from build123d import *

# Parameters (mm, degrees)
SKETCH1_R           = 11.2
BOSS_EXTRUDE1_DEPTH = 232.947291788
CUT_EXTRUDE1_DEPTH  = 236.982


with BuildPart() as part:
    # Sketch1 → Boss-Extrude1 (new body)
    with BuildSketch(Plane.XY):
        with BuildLine():
            Line((-25.4, -67.479999962), (-25.4, 36.365))
            ThreePointArc((-25.4, 36.365), (-23.726115254, 40.406115254), (-19.685, 42.08))
            Line((-19.685, 42.08), (32.385, 42.08))
            ThreePointArc((32.385, 42.08), (36.426115254, 40.406115254), (38.1, 36.365))
            Line((38.1, 36.365), (38.1, 35.095))
            ThreePointArc((38.1, 35.095), (36.426115254, 31.053884746), (32.385, 29.38))
            Line((32.385, 29.38), (-9.652, 29.38))
            ThreePointArc((-9.652, 29.38), (-11.807261469, 28.487261469), (-12.7, 26.332))
            Line((-12.7, 26.332), (-12.7, 22.503))
            ThreePointArc((-12.7, 22.503), (-11.807261469, 20.347738531), (-9.652, 19.455))
            Line((-9.652, 19.455), (0, 19.455))
            Line((0, 19.455), (13.74, 19.455))
            ThreePointArc((13.74, 19.455), (17.781115254, 17.781115254), (19.455, 13.74))
            Line((19.455, 13.74), (19.455, 0))
            Line((19.455, 0), (19.455, -13.74))
            ThreePointArc((19.455, -13.74), (17.781115254, -17.781115254), (13.74, -19.455))
            Line((13.74, -19.455), (0, -19.455))
            Line((0, -19.455), (-9.652, -19.455))
            ThreePointArc((-9.652, -19.455), (-11.807261469, -20.347738531), (-12.7, -22.503))
            Line((-12.7, -22.503), (-12.7, -26.331999962))
            ThreePointArc((-12.7, -26.331999962), (-11.807261469, -28.487261431), (-9.652, -29.379999962))
            Line((-9.652, -29.379999962), (32.385, -29.379999962))
            ThreePointArc((32.385, -29.379999962), (36.426115254, -31.053884708), (38.1, -35.094999962))
            Line((38.1, -35.094999962), (38.1, -67.479999962))
            ThreePointArc((38.1, -67.479999962), (36.240128061, -71.970128023), (31.75, -73.829999962))
            Line((31.75, -73.829999962), (-19.05, -73.829999962))
            ThreePointArc((-19.05, -73.829999962), (-23.540128061, -71.970128023), (-25.4, -67.479999962))
        make_face()
        Circle(SKETCH1_R, mode=Mode.SUBTRACT)
    extrude(amount=BOSS_EXTRUDE1_DEPTH)

    # Sketch2 → Cut-Extrude1 (cut)
    with BuildSketch(Plane.XY.offset(232.947291788)):
        Polygon((19.455, -13.74), (38.1, -13.74), (38.1, 42.08), (19.455, 42.08), (-12.7, 42.08), (-12.7, 22.503), (19.455, 22.503), align=None)
    extrude(amount=-CUT_EXTRUDE1_DEPTH, mode=Mode.SUBTRACT)


solid = part.part
Work out the finished part from the listing and answer in its coordinate system (mm). A direction names the side the tool comes from. Coordinates: 2 decimals unless noted, no trailing zeros. Write each loop counter-clockwise with the first axis right and the second up, starting at its lowest first coordinate (ties: lowest second). Pieces come first, ordered by that corner, then holes. Notation, with made-up numbers: M -36.75,55 L -9.75,55 A16 cw -9.75,67 Z; hole C 40.25,45.5 d4. An arc over 180 degrees is marked long. Write item = value, one per line.
1. The part is cut by section A-A (y = 0). Determine the outline of the cut face in (x, z) (3 decimals).
Solution:
outline = M -25.4,0 L -11.2,0 L -11.2,232.947 L -25.4,232.947 Z; M 11.2,0 L 19.455,0 L 19.455,232.947 L 11.2,232.947 Z
2. For faces 1 (the face through (11, -29.38, 115)), 2 (the face through (19.455, 0, 115)), 3 (the face through (7, -73.83, 115)), determine the directions among +Z, -Z, +X, -X, +Y, -Y from which every point of the face is accessible in a straight line to the end or side of a thin tool.
Solution:
face_1 = +Z, -Z, +X
face_2 = +Z, -Z, +X, +Y
face_3 = +Z, -Z, +X, -X, -Y
3. Determine the mould class of faces 4 (the face through (2, -19.455, 115)), 5 (the face through (-23.77, 40.36, 114.84)), 6 (the face through (36.29, -71.92, 114.84)) for opening direction Y: released by +Y, released by -Y, zero draft, split by the parting line, or undercut.
Solution:
face_4 = undercut
face_5 = released by +Y
face_6 = released by -Y
4. The part is cut by section D-D (y = 32). Determine the outline of the cut face in (x, z).
Solution:
outline = M -25.4,0 L -12.7,0 L -12.7,232.95 L -25.4,232.95 Z
5. Flat-ended cylindrical pins translate along their axes: pin 1 (1 mm diameter, centred on y = -18, z = 119, fed in from +X); pin 2 (3 mm diameter, centred on y = -24, z = 88, fed in from +X); pin 3 (12 mm diameter, centred on x = -1.5, z = 171.5, fed in from +Y) (3 decimals); pin 4 (8 mm diameter, centred on x = 0, y = 26, fed in from +Z). Find the tip coordinate at first contact, or state that the pin passes through.
Solution:
pin_1 = 18.04
pin_2 = -12.7
pin_3 = 19.455
pin_4 = through
6. The part is cut by section C-C (z = 157.5). Determine the outline of the cut face in (x, y) (3 decimals).
Solution:
outline = M -25.4,-67.48 A6.35 ccw -19.05,-73.83 L 31.75,-73.83 A6.35 ccw 38.1,-67.48 L 38.1,-35.095 A5.715 ccw 32.385,-29.38 L -9.652,-29.38 A3.048 cw -12.7,-26.332 L -12.7,-22.503 A3.048 cw -9.652,-19.455 L 13.74,-19.455 A5.715 ccw 19.455,-13.74 L 19.455,13.74 A5.715 ccw 13.74,19.455 L -9.652,19.455 A3.048 cw -12.7,22.503 L -12.7,42.08 L -19.685,42.08 A5.715 ccw -25.4,36.365 Z; hole C 0,0 d22.4
7. The part is cut by section B-B (x = 0). Determine the outline of the cut face in (y, z) (3 decimals), then the cut area to 3 significant figures.
Solution:
outline = M -73.83,0 L -29.38,0 L -29.38,232.947 L -73.83,232.947 Z; M -19.455,0 L -11.2,0 L -11.2,232.947 L -19.455,232.947 Z; M 11.2,0 L 19.455,0 L 19.455,232.947 L 11.2,232.947 Z
area = 14,200 mm2
8. Straight lines are drawn through the part: line 1 (Y direction, x = 0, z = 144) (3 decimals); line 2 (Y direction, x = 4.5, z = 71) (3 decimals); line 3 (X direction, y = 4, z = 21.5) (3 decimals). For each, find the intervals that lie inside material, in ascending order. Write a range as from..to.
Solution:
line_1 = -73.83..-29.38, -19.455..-11.2, 11.2..19.455
line_2 = -73.83..-29.38, -19.455..-10.256, 10.256..19.455
line_3 = -25.4..-10.461, 10.461..19.455
